```python
from build123d import *

# Parameters (mm, degrees)
BOSS_EXTRUDE1_DEPTH           = 18
BOSS_EXTRUDE1_TAPER           = 11
BOSS_EXTRUDE1_OTHER_WAY_DEPTH = 40
BOSS_EXTRUDE1_OTHER_WAY_TAPER = -11
SHELL1_T                      = -2
SKETCH2_W                     = 25
SKETCH2_H                     = 3.2
BOSS_EXTRUDE2_DEPTH           = 20
BOSS_EXTRUDE2_TAPER           = 11


with BuildPart() as part:
    # Sketch1 → Boss-Extrude1 (new body)
    with BuildSketch(Plane(origin=(0, 0, 0), x_dir=(1, 0, 0), z_dir=(0, 1, 0))):
        with BuildLine():
            ThreePointArc((-15, 7.5), (-22.5, 0), (-15, -7.5))
            Line((-15, -7.5), (15, -7.5))
            ThreePointArc((15, -7.5), (22.5, 0), (15, 7.5))
            Line((15, 7.5), (-15, 7.5))
        make_face()
    extrude(amount=-BOSS_EXTRUDE1_DEPTH, taper=BOSS_EXTRUDE1_TAPER)

    # Sketch1 → Boss-Extrude1 other way (add)
    with BuildSketch(Plane(origin=(0, 0, 0), x_dir=(1, 0, 0), z_dir=(0, 1, 0))):
        with BuildLine():
            ThreePointArc((-15, 7.5), (-22.5, 0), (-15, -7.5))
            Line((-15, -7.5), (15, -7.5))
            ThreePointArc((15, -7.5), (22.5, 0), (15, 7.5))
            Line((15, 7.5), (-15, 7.5))
        make_face()
    extrude(amount=BOSS_EXTRUDE1_OTHER_WAY_DEPTH, taper=BOSS_EXTRUDE1_OTHER_WAY_TAPER)

    # Shell1
    shell1_openings = [part.faces().sort_by_distance(p)[0] for p in [
        (0, 40, 0),
        (0, -18, 0),
    ]]
    offset(amount=SHELL1_T, openings=shell1_openings, kind=Kind.INTERSECTION)

    # Sketch2 → Boss-Extrude2 (add)
    with BuildSketch(Plane.XZ.offset(18)):
        with BuildLine():
            ThreePointArc((-15, 4.001154436), (-19.001154436, 0), (-15, -4.001154436))
            Line((-15, -4.001154436), (15, -4.001154436))
            ThreePointArc((15, -4.001154436), (19.001154436, 0), (15, 4.001154436))
            Line((15, 4.001154436), (-15, 4.001154436))
        make_face()
        Rectangle(SKETCH2_W, SKETCH2_H, mode=Mode.SUBTRACT)
    extrude(amount=BOSS_EXTRUDE2_DEPTH, taper=BOSS_EXTRUDE2_TAPER)


solid = part.part
```
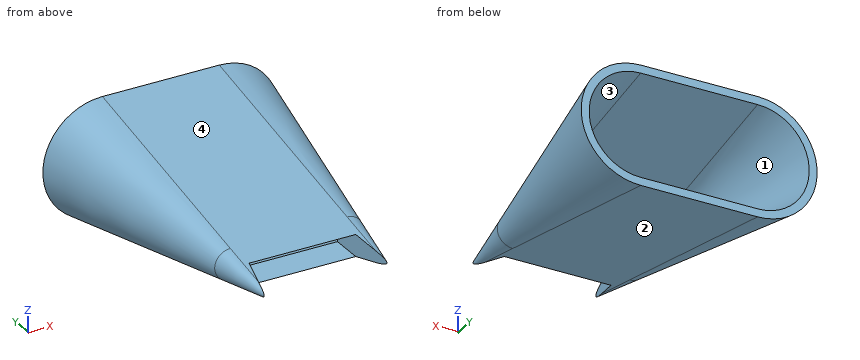
Input: part model. Units: mm. Frame: model coordinates. Face numbers are marked on the shaded views. A direction names the side the tool comes from. Give positions to 0.01 mm unless a question says otherwise; leave off trailing zeros. Loops run counter-clockwise (first coordinate to the right, second up) from the corner with the lowest first, then second, coordinate; pieces in that order, holes last.
1) Line query: L1, parallel to Z at x = -10.5, y = 27; L2, parallel to X at y = 31.5, z = 4; L3, parallel to X at y = 17, z = -4. Output: solid intervals per line, ascending.
A:
L1: z = -12.75 to -10.71, 10.71 to 12.75
L2: x = -28.02 to -25.87, 25.87 to 28.02
L3: x = -25.04 to -22.8, 22.8 to 25.04
2) Section query B-B on y = -10. Return the cut outline in (x, z), and give its area (3 significant figures).
A:
outline: (-15, -5.56) - (15, -5.56) arc R5.56 ccw to (15, 5.56) - (-15, 5.56) arc R5.56 ccw to start; hole (-15, -3.52) - (15, -3.52) arc R3.52 ccw to (15, 3.52) - (-15, 3.52) arc R3.52 ccw to start
area: 180 mm2
3) Reachability of the marked faces 3 and 4 from +Z, -Z, +X, -X, +Y, -Y: full face, straight path, thin tool, end or side. Return the list, or none.
A:
face 3: +Y
face 4: +Z, +X, -X, -Y
4) Mould query, pull axis X, two halves, no side actions, for the marked faces 1 and 2. Classes: released by +X, released by -X, zero draft, split by the parting line, or undercut.
A:
face 1: undercut
face 2: zero draft
5) Section query A-A on y = -2. Return the cut outline in (x, z).
A:
outline: (-15, -7.11) - (15, -7.11) arc R7.11 ccw to (15, 7.11) - (-15, 7.11) arc R7.11 ccw to start; hole (-15, -5.07) - (15, -5.07) arc R5.07 ccw to (15, 5.07) - (-15, 5.07) arc R5.07 ccw to start
6) Contact query for flat-ended pins moving along their axis: pin 1 (2 mm diameter, centred on x = 7, z = 0.5, fed in from +Y); pin 2 (12 mm diameter, centred on x = -8.5, y = 13, fed in from -Z); pin 3 (6 mm diameter, centred on x = 3.5, y = -6.5, fed in from +Z); pin 4 (10 mm diameter, centred on x = 1, y = -14.5, fed in from -Z). Output: stop coordinate, or through.
A:
pin 1: passes through
pin 2: stops at z = -11.19
pin 3: stops at z = 6.82
pin 4: stops at z = -5.65
